Autodesk Fusion 360 part; units mm, degrees
sketch "スケッチ1" plane through (0, 0, 0) normal (0, 0, 1) x (1, 0, 0)
  line L0 (0, -95.5) -> (0, 95.5)
  line L1 (-50, 100) -> (50, 100)
  line L2 (-50, -100) -> (50, -100)
  line L3 (1.15, -95.5) -> (1.15, 95.5)
  line L4 (-1.15, -95.5) -> (-1.15, 95.5)
  line L5 (-50, -95.5) -> (-1.15, -95.5)
  line L6 (1.15, -95.5) -> (50, -95.5)
  line L7 (-50, 95.5) -> (-1.15, 95.5)
  line L8 (1.15, 95.5) -> (50, 95.5)
  line L9 (50, 100) -> (50, 95.5)
  line L10 (-50, 100) -> (-50, 95.5)
  line L11 (-50, -95.5) -> (-50, -100)
  line L12 (50, -95.5) -> (50, -100)
  dimension "d2" = 100
  dimension "d3" = 100
extrude "押し出し1" add sketch "スケッチ1" along normal blind 100
Here's how the part is built. I have some questions about the finished solid (model axes, mm). A direction names the side the tool comes from. Give positions to 0.01 mm unless a question says otherwise; leave off trailing zeros. Order: outer loops, then holes, each group sorted by start corner. A loop starts at its lowest first (then second) coordinate and runs counter-clockwise, first axis right, second up. Notation, with made-up numbers: (-7, 6.25) - (-3, 6.25) arc R10 cw to (-3, 22.25) - close; hole circle Ø6 at (82.25, 7.5). An arc over 180 degrees is marked (long way). Answer as a JSON object with one key per item and string values. Group by question number.
Item 1: If we section it at C-C on y = -72: Please give me the cut outline in (x, z).
Item 2: Which directions (+Z, -Z, +X, -X, +Y, -Y) give clear straight access to the entire face, cutting with the end or side of a thin tool? Please do faces 4 (the flat face through (50, 98, 49)), 5 (the flat face through (-26, -95.5, 49)), 6 (the flat face through (25, -95.5, 49)).
Item 3: If we mould it in two halves opening along Y, with no side actions, what happens to faces 1 (the flat face through (-1, 100, 49)), 2 (the flat face through (1.15, -1, 49)), 3 (the flat face through (-50, 98, 49))? For each: pulls with the +Y half, pulls with the -Y half, needs draft (parallel to the pull), parting line crosses it, or undercut.
Item 4: For P1, Ø3, axis at y = 26.5, z = 76, coming from the -X side; P2, Ø3, axis at y = 65, z = 80.5, coming from the +X side, each with a flat end and sliding along its axis, tell me the tip position at first contact or that it passes through.
Item 5: If we section it at B-B on z = 44: Please give me the cut outline in (x, y).
Item 6: Please list where these lines run through material, in increasing order: probe 1 along Y at (x, z) = (-44, 72); probe 2 along X at (y, z) = (81.5, 29.5).
Item 7: If we section it at A-A on x = 23: Please give me the cut outline in (y, z), and give its area (3 significant figures).
Result set:
{
 "1": {"outline": "(-1.15, 0) - (1.15, 0) - (1.15, 100) - (-1.15, 100) - close"},
 "2": {"face 4": "+Z, -Z, +X, +Y, -Y", "face 5": "+Z, -Z, -X", "face 6": "+Z, -Z, +X"},
 "3": {"face 1": "pulls with the +Y half", "face 2": "undercut", "face 3": "needs draft"},
 "4": {"P1": "x = -1.15", "P2": "x = 1.15"},
 "5": {"outline": "(-50, -100) - (50, -100) - (50, -95.5) - (1.15, -95.5) - (1.15, 95.5) - (50, 95.5) - (50, 100) - (-50, 100) - (-50, 95.5) - (-1.15, 95.5) - (-1.15, -95.5) - (-50, -95.5) - close"},
 "6": {"probe 1": "-100 to -95.5, 95.5 to 100", "probe 2": "-1.15 to 1.15"},
 "7": {"outline": "(-100, 0) - (-95.5, 0) - (-95.5, 100) - (-100, 100) - close; (95.5, 0) - (100, 0) - (100, 100) - (95.5, 100) - close", "area": "900 mm²"}
}
